```python
from build123d import *

# Parameters (mm, degrees)
SKETCH1_R           = 1.575
BOSS_EXTRUDE1_DEPTH = 5
SKETCH2_R           = 3.928649494
CUT_EXTRUDE1_DEPTH  = 3


with BuildPart() as part:
    # Sketch1 → Boss-Extrude1 (new, symmetric)
    with BuildSketch(Plane.XY):
        with BuildLine():
            Line((9.732479224, 4.807479224), (9.732479224, 9.557479224))
            ThreePointArc((9.732479224, 9.557479224), (9.539846423, 10.964172818), (8.976131504, 12.267292058))
            Line((8.976131504, 12.267292058), (5.455637648, 18.08252522))
            ThreePointArc((5.455637648, 18.08252522), (2.532334022, 19.240369543), (0.631218006, 16.735960338))
            Line((0.631218006, 16.735960338), (0.631218006, 13.950074632))
            Line((0.631218006, 13.950074632), (1.131218006, 13.950074632))
            Line((1.131218006, 13.950074632), (2.83470481, 15.653561435))
            Line((2.83470481, 15.653561435), (5.98205172, 10.454701026))
            ThreePointArc((5.98205172, 10.454701026), (6.168698307, 10.023236912), (6.232479224, 9.557479224))
            Line((6.232479224, 9.557479224), (6.232479224, 4.807479224))
            ThreePointArc((6.232479224, 4.807479224), (5.725047808, 3.582431417), (4.5, 3.075))
            Line((4.5, 3.075), (0, 3.075))
            ThreePointArc((0, 3.075), (-2.840929562, 1.176751555), (-2.174353352, -2.174353352))
            Line((-2.174353352, -2.174353352), (1.517126313, -5.865833018))
            ThreePointArc((1.517126313, -5.865833018), (4.042707088, -6.11440715), (4.778890142, -3.685748701))
            ThreePointArc((4.778890142, -3.685748701), (4.653279573, -2.058204966), (5.513269646, -0.670727508))
            Line((5.513269646, -0.670727508), (8.260484532, 1.643135904))
            ThreePointArc((8.260484532, 1.643135904), (9.346473058, 3.062498062), (9.732479224, 4.807479224))
        make_face()
        Circle(SKETCH1_R, mode=Mode.SUBTRACT)
    extrude(amount=BOSS_EXTRUDE1_DEPTH, both=True)

    # Sketch2 → Cut-Extrude1 (cut, symmetric)
    with BuildSketch(Plane.XY):
        Circle(SKETCH2_R)
    extrude(amount=CUT_EXTRUDE1_DEPTH, both=True, mode=Mode.SUBTRACT)


solid = part.part
```
Geometry check sheet. Reference: the model listing, model coordinates, mm. A direction names the side the tool comes from. Coordinates: 2 decimals unless noted, no trailing zeros. Order: outer loops, then holes, each group sorted by start corner. A loop starts at its lowest first (then second) coordinate and runs counter-clockwise, first axis right, second up. Notation, with made-up numbers: M 38,12 L 82,12 A18 ccw 82,39 Z; hole C 49.5,-3.5 d7. An arc over 180 degrees is marked long. One line per question, with ' | ' between items. Start each with the question number.
Item 1: Set-up check for faces 1 (the cylindrical face through (4.65, -2.08, 0.07)), 2 (the flat face through (6.232, 7, 0)), 3 (the flat face through (4.386, 13.091, 0.07)): record each of +Z, -Z, +X, -X, +Y, -Y from which the full face is reachable in a straight line by a thin tool's end or side.
Item 2: Cross-section at A-A on x = -1. Enter the section's corners in (y, z).
Item 3: Cross-section at D-D on y = 6.25. Enter the section's corners in (x, z), then the cut area to 3 significant figures.
Item 4: Draft check along Y on faces 4 (the cylindrical face through (-2.821, 1.223, 4.014)), 5 (the flat face through (1.97, 14.79, 0.07)), 6 (the cylindrical face through (9.545, 10.945, 0.07)). Enter one of: pulls with the +Y half, pulls with the -Y half, needs draft (parallel to the pull), parting line crosses it, or undercut.
Item 5: Cross-section at C-C on y = 0. Enter the section's corners in (x, z) (3 decimals).
Item 6: Cross-section at B-B on z = 4.25. Enter the section's corners in (x, y) (3 decimals).
Item 7: Material ranges on L1, parallel to Y at x = 6, z = 1.5; L2, parallel to Y at x = 0, z = -3.45 (3 decimals); L3, parallel to X at y = 0, z = 3.55 (3 decimals), recorded low to high. Write a range as [from, to].
Item 8: Gauge pin test, flat ends, axial feed: pin 1 (2.5 mm diameter, centred on x = 0, y = 0, fed in from +Z); pin 2 (4 mm diameter, centred on y = 8, z = -3.5, fed in from -X) (3 decimals); pin 3 (3 mm diameter, centred on x = 1, z = -3, fed in from -Y); pin 4 (2 mm diameter, centred on y = 14.5, z = 1, fed in from -X). Record the tip position at first contact, or that the pin passes through.
Findings:
1) face 1: +Z, -Z, +X | face 2: +Z, -Z, -X | face 3: +Z, -Z
2) outline: M -3.35,-5 L -1.22,-5 L -1.22,-3 L -3.35,-3 Z; M -3.35,3 L -1.22,3 L -1.22,5 L -3.35,5 Z; M 1.22,-5 L 2.91,-5 L 2.91,-3 L 1.22,-3 Z; M 1.22,3 L 2.91,3 L 2.91,5 L 1.22,5 Z
3) outline: M 6.23,-5 L 9.73,-5 L 9.73,5 L 6.23,5 Z | area: 35.0 mm²
4) face 4: parting line crosses it | face 5: undercut | face 6: pulls with the +Y half
5) outline: M -3.075,-5 L -1.575,-5 L -1.575,-3 L -3.075,-3 Z; M -3.075,3 L -1.575,3 L -1.575,5 L -3.075,5 Z; M 1.575,-5 L 6.31,-5 L 6.31,5 L 1.575,5 L 1.575,3 L 3.929,3 L 3.929,-3 L 1.575,-3 Z
6) outline: M -2.174,-2.174 L 1.517,-5.866 A2 ccw 4.779,-3.686 A2.627 cw 5.513,-0.671 L 8.26,1.643 A4.137 ccw 9.732,4.807 L 9.732,9.557 A5.232 ccw 8.976,12.267 L 5.456,18.083 A2.6 ccw 0.631,16.736 L 0.631,13.95 L 1.131,13.95 L 2.835,15.654 L 5.982,10.455 A1.732 cw 6.232,9.557 L 6.232,4.807 A1.732 cw 4.5,3.075 L 0,3.075 A3.075 ccw Z; hole C 0,0 d3.15
7) L1: y = [-0.26, 3.94], [10.42, 17.18] | L2: y = [-4.349, -1.575], [1.575, 3.075] | L3: x = [-3.075, -1.575], [1.575, 6.31]
8) pin 1: passes through | pin 2: stops at x = 6.175 | pin 3: stops at y = -6.4 | pin 4: stops at x = 0.63
